Model file for the job. Use its own axes, mm. A direction names the side the tool comes from. Round coordinates to 2 decimals unless told otherwise and drop trailing zeros. Order: outer loops, then holes, each group sorted by start corner. A loop starts at its lowest first (then second) coordinate and runs counter-clockwise, first axis right, second up. Notation, with made-up numbers: (22.5, 61) - (48.5, 61) arc R17 ccw to (48.5, 67) - close; hole circle Ø2 at (10, 50). An arc over 180 degrees is marked (long way). Answer as CSV lines item,"result". Start each with the question number.
1. 3-axis set-ups, long thin cutter, end or side, ignore diameter. For faces 1 (the face through (0, 18, 6)), 2 (the face through (-7, 0, 10)), 3 (the face through (-2, -1.56, 10)), 4 (the face through (7, 0, 10)): which of +Z, -Z, +X, -X, +Y, -Y reach the whole face in a straight line?
2. Pull direction Y, two halves, no side cores. Call faces 5 (the face through (3.83, -0.79, 9.86)), 6 (the face through (-0.534, 29.965, 2.958)), 7 (the face through (-9.014, 17.963, 12.902)), 8 (the face through (10, 13, 8)): released by +Y, released by -Y, zero draft, split by the parting line, or undercut.
3. Band-saw the part on D-D on y = 24. List the corners of the cut face in (x, z).
4. Wall check: line 1 along Z through (x, y) = (0, 1.4); line 2 along Y through (x, z) = (0, 3.05); line 3 along X through (y, z) = (6, 15.5). Give the ranges that are in metal, low to high. Write a range as [from, to].
5. Pin check, flat tips, straight feed: pin 1 Ø8 at (x, z) = (5.5, 4) entering from -Y; pin 2 Ø3 at (x, z) = (0, 10) entering from -Y; pin 3 Ø2.5 at (x, z) = (-6.5, 12) entering from -Y; pin 4 Ø8 at (x, y) = (0, 18.5) entering from +Z. Stop position of each tip, or through.
6. Band-saw the part on B-B on z = 4. List the corners of the cut face in (x, y).
7. Band-saw the part on A-A on x = 0. List the corners of the cut face in (y, z).
8. Band-saw the part on C-C on x = 2.5. List the corners of the cut face in (y, z).
```python
from build123d import *

# Parameters (mm, degrees)
SKETCH_R            = 4.1
PAD_DEPTH           = 6
SKETCH001_W         = 2.5
SKETCH001_H         = 14
PAD001_DEPTH        = 20
PAD002_DEPTH        = 14
PAD003_DEPTH        = 2
LINEARPATTERN_COUNT = 2
LINEARPATTERN_PITCH = 18
SKETCH003_R         = 1.6
POCKET_DEPTH        = 34.561


with BuildPart() as part:
    # Sketch → Pad (new body)
    with BuildSketch(Plane.XY):
        Polygon((-4.74, 0), (-2.94, -1.56), (2.94, -1.56), (4.74, 0), (10, 0), (10, 33), (-10, 33), (-10, 0), align=None)
        with Locations((0, 25.9)):
            Circle(SKETCH_R, mode=Mode.SUBTRACT)
    extrude(amount=PAD_DEPTH)

    # Sketch001 (on Face5 of Pad) → Pad001 (join)
    with BuildSketch(Plane.YZ.offset(10)):
        with Locations((1.25, 13)):
            Rectangle(SKETCH001_W, SKETCH001_H)
    extrude(amount=-PAD001_DEPTH)

    # Pad001 Face5 → Pad002 (add)
    with BuildSketch(Plane(origin=(0, -0.719062, 6), x_dir=(0, 1, 0), z_dir=(0, 0, 1))):
        Polygon((0.719062, -4.74), (0.719062, 4.74), (-0.840938, 2.94), (-0.840938, -2.94), align=None)
    extrude(amount=PAD002_DEPTH)

    # Sketch002 (on Face6 of Pad002) → Pad003 (join)
    with BuildSketch(Plane(origin=(-10, 0, 0), x_dir=(0, -1, 0), z_dir=(-1, 0, 0))):
        Polygon((-33, 6), (-2.5, 20), (-2.5, 6), align=None)
    pad003 = extrude(amount=-PAD003_DEPTH)

    # LinearPattern: Pad003 ×2
    with Locations(*[(i * LINEARPATTERN_PITCH, 0, 0) for i in range(1, LINEARPATTERN_COUNT)]):
        add(pad003)

    # Sketch003 (on Face9 of LinearPattern) → Pocket (cut, through all)
    with BuildSketch(Plane.XZ.offset(1.56)):
        with Locations((0, 10)):
            Circle(SKETCH003_R)
    extrude(amount=-POCKET_DEPTH, mode=Mode.SUBTRACT)


solid = part.part
```
Reply:
1,face 1,"+Z, +Y"
1,face 2,"+Z, -Z, -X, -Y"
1,face 3,"+Z, -Z, +X, -X, -Y"
1,face 4,"+Z, -Z, +X, -Y"
2,face 5,"released by -Y"
2,face 6,"undercut"
2,face 7,"released by +Y"
2,face 8,"zero draft"
3,outline,"(-10, 0) - (-3.63, 0) - (-3.63, 6) - (-8, 6) - (-8, 10.13) - (-10, 10.13) - close; (3.63, 0) - (10, 0) - (10, 10.13) - (8, 10.13) - (8, 6) - (3.63, 6) - close"
4,line 1,"z = [0, 8.4], [11.6, 20]"
4,line 2,"y = [-1.56, 21.8], [30, 33]"
4,line 3,"x = [-10, -8], [8, 10]"
5,pin 1,"stops at y = -1.56"
5,pin 2,"passes through"
5,pin 3,"stops at y = 0"
5,pin 4,"stops at z = 6"
6,outline,"(-10, 0) - (-4.74, 0) - (-2.94, -1.56) - (2.94, -1.56) - (4.74, 0) - (10, 0) - (10, 33) - (-10, 33) - close; hole circle Ø8.2 at (0, 25.9)"
7,outline,"(-1.56, 0) - (21.8, 0) - (21.8, 6) - (2.5, 6) - (2.5, 8.4) - (-1.56, 8.4) - close; (-1.56, 11.6) - (2.5, 11.6) - (2.5, 20) - (-1.56, 20) - close; (30, 0) - (33, 0) - (33, 6) - (30, 6) - close"
8,outline,"(-1.56, 0) - (22.65, 0) - (22.65, 6) - (2.5, 6) - (2.5, 20) - (-1.56, 20) - close; (29.15, 0) - (33, 0) - (33, 6) - (29.15, 6) - close"
